Could you check a few things on this model? Use its own coordinates, in mm. A direction names the side the tool comes from. Round coordinates to 2 decimals unless told otherwise and drop trailing zeros. Write each loop counter-clockwise with the first axis right and the second up, starting at its lowest first coordinate (ties: lowest second). Pieces come first, ordered by that corner, then holes. Notation, with made-up numbers: M -14,-31.5 L 25,-31.5 A16 ccw 25,-16.5 Z; hole C -11,9 d1. An arc over 180 degrees is marked long. One line per question, with ' | ' between items. Start each with the question number.
```python
from build123d import *

# Parameters (mm, degrees)
SKETCH2_W            = 15.94
SKETCH2_H            = 21.4
BOSS_EXTRUDE1_DEPTH  = 13.5
CUT_EXTRUDE1_DEPTH   = 8.56
CHAMFER1_SIZE        = 0.5
SKETCH4_W            = 3.71
SKETCH4_H            = 1.73
CUT_EXTRUDE2_DEPTH   = 8
BOSS_EXTRUDE2_DEPTH  = 8
BOSS_EXTRUDE5_DEPTH  = 0.25
LPATTERN1_COUNT      = 8
LPATTERN1_PITCH      = 1
BOSS_EXTRUDE7_START  = 7.97
BOSS_EXTRUDE7_DEPTH  = 0.4
BOSS_EXTRUDE8_START  = -7.97
BOSS_EXTRUDE8_DEPTH  = 0.4
SKETCH9_R            = 1.625
BOSS_EXTRUDE9_DEPTH  = 3
CUT_EXTRUDE3_DEPTH   = 3
CHAMFER2_SIZE        = 0.3
SKETCH11_R           = 0.445
BOSS_EXTRUDE10_DEPTH = 3
CHAMFER3_SIZE        = 0.15


with BuildPart() as part:
    # Sketch2 → Boss-Extrude1 (new body)
    with BuildSketch(Plane(origin=(0, 0, 0), x_dir=(1, 0, 0), z_dir=(0, 1, 0))):
        Rectangle(SKETCH2_W, SKETCH2_H)
    extrude(amount=BOSS_EXTRUDE1_DEPTH)

    # Sketch3 → Cut-Extrude1 (cut)
    with BuildSketch(Plane.XY.offset(10.7)):
        Polygon((-5.97, 10.81), (5.97, 10.81), (5.97, 2.81), (2.87, 2.81), (2.87, 1.51), (1.91, 1.51), (1.91, 0.81), (-1.91, 0.81), (-1.91, 1.51), (-2.87, 1.51), (-2.87, 2.81), (-5.97, 2.81), align=None)
    extrude(amount=-CUT_EXTRUDE1_DEPTH, mode=Mode.SUBTRACT)

    # Chamfer1
    chamfer1_edges = [part.edges().sort_by_distance(p)[0] for p in [
        (-5.97, 6.81, 10.7),
        (-4.42, 2.81, 10.7),
        (-2.87, 2.16, 10.7),
        (-2.39, 1.51, 10.7),
        (-1.91, 1.16, 10.7),
        (0, 0.81, 10.7),
        (1.91, 1.16, 10.7),
        (2.39, 1.51, 10.7),
        (2.87, 2.16, 10.7),
        (4.42, 2.81, 10.7),
        (5.97, 6.81, 10.7),
        (0, 10.81, 10.7),
    ]]
    chamfer(chamfer1_edges, length=CHAMFER1_SIZE)

    # Sketch4 → Cut-Extrude2 (cut)
    with BuildSketch(Plane.XY.offset(10.7)):
        with Locations((-5.525, 1.145)):
            Rectangle(SKETCH4_W, SKETCH4_H)
        with Locations((5.525, 1.145)):
            Rectangle(SKETCH4_W, SKETCH4_H)
    extrude(amount=-CUT_EXTRUDE2_DEPTH, mode=Mode.SUBTRACT)

    # Sketch5 → Boss-Extrude2 (add)
    with BuildSketch(Plane.XY.offset(2.7)):
        with BuildLine():
            Line((-7.13, 1.96), (-3.92, 1.96))
            ThreePointArc((-3.92, 1.96), (-3.778578644, 1.901421356), (-3.72, 1.76))
            Line((-3.72, 1.76), (-3.72, 0.53))
            ThreePointArc((-3.72, 0.53), (-3.778578644, 0.388578644), (-3.92, 0.33))
            Line((-3.92, 0.33), (-7.13, 0.33))
            ThreePointArc((-7.13, 0.33), (-7.271421356, 0.388578644), (-7.33, 0.53))
            Line((-7.33, 0.53), (-7.33, 1.76))
            ThreePointArc((-7.33, 1.76), (-7.271421356, 1.901421356), (-7.13, 1.96))
        make_face()
        with BuildLine():
            Line((3.72, 1.76), (3.72, 0.53))
            ThreePointArc((3.72, 0.53), (3.778578644, 0.388578644), (3.92, 0.33))
            Line((3.92, 0.33), (7.13, 0.33))
            ThreePointArc((7.13, 0.33), (7.271421356, 0.388578644), (7.33, 0.53))
            Line((7.33, 0.53), (7.33, 1.76))
            ThreePointArc((7.33, 1.76), (7.271421356, 1.901421356), (7.13, 1.96))
            Line((7.13, 1.96), (3.92, 1.96))
            ThreePointArc((3.92, 1.96), (3.778578644, 1.901421356), (3.72, 1.76))
        make_face()
    extrude(amount=BOSS_EXTRUDE2_DEPTH)

    # Sketch6 → Boss-Extrude5 (add, symmetric)
    with BuildSketch(Plane.ZY.offset(-3.47)):
        with BuildLine():
            Line((9.157258215, 10.804234071), (9.157258215, 10.623877591))
            ThreePointArc((9.157258215, 10.623877591), (9.087595817, 10.431667837), (8.910960953, 10.328723367))
            Line((8.910960953, 10.328723367), (2.14, 9.096760174))
            Line((2.14, 9.096760174), (2.14, 9.52745757))
            Line((2.14, 9.52745757), (9.157258215, 10.804234071))
        make_face()
    boss_extrude5 = extrude(amount=BOSS_EXTRUDE5_DEPTH, both=True)

    # LPattern1: Boss-Extrude5 ×8
    with Locations(*[(-i * LPATTERN1_PITCH, 0, 0) for i in range(1, LPATTERN1_COUNT)]):
        add(boss_extrude5)

    # Sketch8 → Boss-Extrude7 (add)
    with BuildSketch(Plane(origin=(0, 0, 0), x_dir=(0, 0, -1), z_dir=(1, 0, 0)).offset(BOSS_EXTRUDE7_START)):
        with BuildLine():
            Line((4.02, 0), (4.02, -2.25))
            ThreePointArc((4.02, -2.25), (3.27, -3), (2.52, -2.25))
            Line((2.52, -2.25), (2.52, 0))
            Line((2.52, 0), (4.02, 0))
        make_face()
    extrude(amount=-BOSS_EXTRUDE7_DEPTH)

    # Sketch8_2 → Boss-Extrude8 (add)
    with BuildSketch(Plane(origin=(0, 0, 0), x_dir=(0, 0, -1), z_dir=(1, 0, 0)).offset(BOSS_EXTRUDE8_START)):
        with BuildLine():
            Line((4.02, 0), (4.02, -2.25))
            ThreePointArc((4.02, -2.25), (3.27, -3), (2.52, -2.25))
            Line((2.52, -2.25), (2.52, 0))
            Line((2.52, 0), (4.02, 0))
        make_face()
    extrude(amount=BOSS_EXTRUDE8_DEPTH)

    # Sketch9 → Boss-Extrude9 (add)
    with BuildSketch(Plane.XZ):
        with Locations((6.030646147, -0.22)):
            Circle(SKETCH9_R)
        with Locations((-6.030646147, -0.22)):
            Circle(SKETCH9_R)
    extrude(amount=BOSS_EXTRUDE9_DEPTH)

    # Sketch10 → Cut-Extrude3 (cut)
    with BuildSketch(Plane.XZ):
        with BuildLine():
            ThreePointArc((-5.673759882, 1.36532558), (-6.030646147, 1.405), (-6.387532412, 1.36532558))
            Line((-6.387532412, 1.36532558), (-6.387532412, -1.80532558))
            ThreePointArc((-6.387532412, -1.80532558), (-6.030646147, -1.845), (-5.673759882, -1.80532558))
            Line((-5.673759882, -1.80532558), (-5.673759882, 1.36532558))
        make_face()
        with BuildLine():
            ThreePointArc((6.387532412, 1.36532558), (6.030646147, 1.405), (5.673759882, 1.36532558))
            Line((5.673759882, 1.36532558), (5.673759882, -1.80532558))
            ThreePointArc((5.673759882, -1.80532558), (6.030646147, -1.845), (6.387532412, -1.80532558))
            Line((6.387532412, -1.80532558), (6.387532412, 1.36532558))
        make_face()
    extrude(amount=CUT_EXTRUDE3_DEPTH, mode=Mode.SUBTRACT)

    # Chamfer2
    chamfer2_edges = [part.edges().sort_by_distance(p)[0] for p in [
        (4.405646147, -3, -0.22),
        (-4.405646147, -3, -0.22),
        (-7.655646147, -3, -0.22),
        (7.655646147, -3, -0.22),
    ]]
    chamfer(chamfer2_edges, length=CHAMFER2_SIZE)

    # Sketch11 → Boss-Extrude10 (add)
    with BuildSketch(Plane.XZ):
        with Locations((-5.013424508, -9.11)):
            Circle(SKETCH11_R)
        with Locations((-2.473424508, -9.11)):
            Circle(SKETCH11_R)
        with Locations((0.066575492, -9.11)):
            Circle(SKETCH11_R)
        with Locations((2.606575492, -9.11)):
            Circle(SKETCH11_R)
        with Locations((-3.719101646, -6.57)):
            Circle(SKETCH11_R)
        with Locations((-1.179101646, -6.57)):
            Circle(SKETCH11_R)
        with Locations((1.360898354, -6.57)):
            Circle(SKETCH11_R)
        with Locations((3.900898354, -6.57)):
            Circle(SKETCH11_R)
    extrude(amount=BOSS_EXTRUDE10_DEPTH)

    # Chamfer3
    chamfer3_edges = [part.edges().sort_by_distance(p)[0] for p in [
        (-5.458424508, -3, -9.11),
        (-2.918424508, -3, -9.11),
        (-0.378424508, -3, -9.11),
        (2.161575492, -3, -9.11),
        (-4.164101646, -3, -6.57),
        (-1.624101646, -3, -6.57),
        (0.915898354, -3, -6.57),
        (3.455898354, -3, -6.57),
    ]]
    chamfer(chamfer3_edges, length=CHAMFER3_SIZE)


solid = part.part
```
1. I need wall thicknesses on line 1 along Y through (x, z) = (1.75, 7); line 2 along X through (y, z) = (-0.5, 0.5); line 3 along Y through (x, z) = (-2.75, 7.5). Which ranges of each line are inside material? Lowest first, please. Write a range as from..to.
2. Suppose I cut it at D-D (z = -3.27). Write out the boundary of the cut face in (x, y), and give its area (3 significant figures).
3. If we mould it in two halves opening along Z, with no side actions, what happens to faces 6 (the face through (2.51, -1.405, -9.544)), 7 (the face through (0, 0.81, 6)), 8 (the face through (-3.533, 10.157, 5.6))? For each: released by +Z, released by -Z, zero draft, split by the parting line, or undercut.
4. Which directions (+Z, -Z, +X, -X, +Y, -Y) give clear straight access to the entire face, cutting with the end or side of a thin tool? Please do faces 1 (the face through (-2.78, 10, 6)), 2 (the face through (-4.406, -1.331, -0.251)), 3 (the face through (-7, -3, 0)), 4 (the face through (-7.655, -1.331, -0.189)), 5 (the face through (0, 13.5, 0)).
5. Suppose I cut it at C-C (z = 5.25). Count the separate pieces of the cut face and the enclosed holes in it, and give its area (3 significant figures).
6. I'm going to push flat-ended pins straight in: P1, Ø1.5, axis at x = 3, z = 6.5, coming from the -Y side; P2, Ø1, axis at x = 3, y = 6.5, coming from the +Z side; P3, Ø2.5, axis at y = -1.5, z = 0.5, coming from the -X side. Where does each tip first touch, or does it pass through?
7. Suppose I cut it at B-B (y = 8.5). Write out the boundary of the cut face in (x, z), and give its area (3 significant figures).
8. Suppose I cut it at A-A (z = -6.57). Write out the boundary of the cut face in (x, y), and give its area (3 significant figures).
Computed:
1) line 1: y = 0..0.81, 10.81..13.5 | line 2: x = -7.49..-6.39, -5.67..-4.57, 4.57..5.67, 6.39..7.49 | line 3: y = 0..1.51, 10.07..10.5, 10.81..13.5
2) outline: M -7.97,-3 L -7.57,-3 L -7.57,0 L 7.57,0 L 7.57,-3 L 7.97,-3 L 7.97,13.5 L -7.97,13.5 Z | area: 218 mm²
3) face 6: split by the parting line | face 7: zero draft | face 8: undercut
4) face 1: +Z | face 2: -Y | face 3: +Z, -Z, +X, -X, -Y | face 4: -X, -Y | face 5: +Z, -Z, +X, -X, +Y
5) separate pieces: 11 | enclosed holes: 3 | area: 110 mm²
6) P1: stops at y = 0 | P2: stops at z = 2.14 | P3: stops at x = -7.66
7) outline: M -7.97,-10.7 L 7.97,-10.7 L 7.97,10.7 L 6.47,10.7 L 5.97,10.2 L 5.97,2.14 L -5.97,2.14 L -5.97,10.2 L -6.47,10.7 L -7.97,10.7 Z | area: 239 mm²
8) outline: M -7.97,0 L -4.16,0 L -4.16,-2.85 L -4.01,-3 L -3.42,-3 L -3.27,-2.85 L -3.27,0 L -1.62,0 L -1.62,-2.85 L -1.47,-3 L -0.88,-3 L -0.73,-2.85 L -0.73,0 L 0.92,0 L 0.92,-2.85 L 1.07,-3 L 1.66,-3 L 1.81,-2.85 L 1.81,0 L 3.46,0 L 3.46,-2.85 L 3.61,-3 L 4.2,-3 L 4.35,-2.85 L 4.35,0 L 7.97,0 L 7.97,13.5 L -7.97,13.5 Z | area: 226 mm²
